Check sheet for the modelled part. Datum: model origin and axes. Units: mm. A direction names the side the tool comes from. Round coordinates to 2 decimals unless told otherwise and drop trailing zeros. Order: outer loops, then holes, each group sorted by start corner. A loop starts at its lowest first (then second) coordinate and runs counter-clockwise, first axis right, second up. Notation, with made-up numbers: M 79.25,47.5 L 87.25,47.5 A11 cw 87.25,63.5 Z; hole C -28.5,36.25 d11. An arc over 180 degrees is marked long. One line per item, written item: value. Start each with the question number.
(1) Thickness scan on L1, parallel to Y at x = -12, z = -41.5; L2, parallel to X at y = 4, z = -9.5; L3, parallel to X at y = 4.75, z = -39. Record the ranges inside material, lowest first.
(2) Release check for a two-part mould opening along X. For faces 4 (the face through (0, 5, -36)), 5 (the face through (-12.14, 4.01, -39.58)), 6 (the face through (-13.52, 4.93, -37.37)) record: released by +X, released by -X, zero draft, split by the parting line, or undercut.
(3) Depth check by flat-ended pin: pin 1 Ø5 at (x, y) = (-32, 4) entering from -Z. Enter the tip coordinate at first touch or a pass-through.
(4) Cross-section at D-D, the plane z = -28. Enter the section's corners in (x, y).
(5) Access from +Z, -Z, +X, -X, +Y, -Y to the whole of each face (thin tool, end or side, straight path). Record for faces 1 (the face through (-5.07, 4.93, -43.996)), 2 (the face through (-26.128, 5, -8)), 3 (the face through (-9.24, 5.04, -40.69)).
(6) Cross-section at C-C, the plane x = -28.5. Enter the section's corners in (y, z).
(7) Cross-section at A-A, the plane x = -6. Enter the section's corners in (y, z), and give its area (3 significant figures).
Autodesk Inventor part; units mm, degrees
ref_plane "YZ Plane" through (0, 0, 0) normal (1, 0, 0) x (0, 1, 0)
ref_plane "XZ Plane" through (0, 0, 0) normal (0, 1, 0) x (-1, 0, 0)
ref_plane "XY Plane" through (0, 0, 0) normal (0, 0, 1) x (1, 0, 0)
sketch "Sketch1" plane through (0, 0, 0) normal (0, 1, 0) x (-1, 0, 0)
  line L0 (36.1277, -22.2455) -> (12, -36.4736)
  line L1 (12, -36.4736) -> (15.0796, -38.2896)
  line L2 (15.0796, -38.2896) -> (10, -46.9035)
  line L3 (10, -46.9035) -> (0, -41.0064)
  line L4 (36.1277, -22.2455) -> (36.1277, 0)
  line L5 (36.1277, 0) -> (26.1277, 0)
  line L6 (26.1277, 0) -> (26.1277, -16.5333)
  line L7 (26.1277, -16.5333) -> (0, -31.9408)
  line L8 (0, -31.9408) -> (0, -41.0064)
  line L9 (0, -36.4736) -> (12, -36.4736) construction
  circle A0 centre (6, -36.4736) radius 3.175
  point P0 (0, 0)
  dimension "d1" = 10
  dimension "d8" = 10
  dimension "d9" = 10
  dimension "d10" = 10
  dimension "d12" = 12
  dimension "d13" = 6.35
  dimension "d14" = 22.2455
  dimension "d17" = 61.056
  dimension "d19" = 28.0104
extrude "Extrusion1" add sketch "Sketch1" along normal blind 10
sketch "Sketch2" plane through (-15.0796, 0, -38.2896) normal (-0.8613822, 0, -0.5079575) x (-0.5079575, 0, 0.8613822)
  line L0 (0, 0) -> (-10, 0)
  line L1 (0, 0) -> (0, 10)
  line L2 (-10, 10) -> (0, 10)
  line L3 (-10, 0) -> (-10, 10)
  line L4 (-5, 10) -> (-5, 0) construction
  line L5 (-10, 5) -> (-5, 5) construction
  circle A0 centre (-5, 5) radius 2.5275
  circle A1 centre (-5, 5) radius 2.6545
  point P0 (25.3222, 0)
  dimension "d22" = 5.055
  dimension "d23" = 5.309
extrude "Extrusion2" cut sketch "Sketch2" against normal blind 3.81 contours A0
sketch "Sketch3" plane through (-9.2579, 5, -40.6612) normal (-0.8613822, 0, -0.5079575) x (-0.5079575, 0, 0.8613822)
  line L0 (-5, 0) -> (0, 0) construction
  circle A0 centre (0, 0) radius 2.5275
  circle A1 centre (0, 0) radius 2.5275
  point P0 (30.3222, -5)
loft "Loft1" cut profiles "Sketch2" section 2 edges at (-7.9723, 5, -42.8373) contours A0 | A1
properties part number "seeSaw"
Values found:
1. L1: 0 to 2.47, 7.53 to 10
1. L2: -36.13 to -26.13
1. L3: -14.66 to -11.46, -10.24 to -7.92, -4.08 to 0
2. face 4: released by +X
2. face 5: undercut
2. face 6: released by -X
3. pin 1: z = -26.15
4. outline: M -26.37,0 L -6.68,0 L -6.68,10 L -26.37,10 Z
5. face 1: -Z, +X, +Y, -Y
5. face 2: +Z, +X, +Y, -Y
5. face 3: none
6. outline: M 0,-26.74 L 10,-26.74 L 10,0 L 0,0 Z
7. outline: M 0,-44.54 L 10,-44.54 L 10,-39.65 L 0,-39.65 Z; M 0,-33.3 L 10,-33.3 L 10,-28.4 L 0,-28.4 Z
7. area: 97.9 mm^2
